Could you check a few things on this model? Use its own coordinates, in mm. Face numbers are marked on the shaded views. Give positions to 0.01 mm unless a question says otherwise; leave off trailing zeros. Write each loop counter-clockwise with the first axis right and the second up, starting at its lowest first coordinate (ties: lowest second). Pieces come first, ordered by that corner, then holes. Notation, with made-up numbers: (-37.5, 78.5) -> (-19.5, 78.5) arc R31 cw to (-19.5, 115.5) -> close; hole circle Ø11 at (-39, 36). An arc over 180 degrees is marked (long way). One line per question, with ' | ' between items.
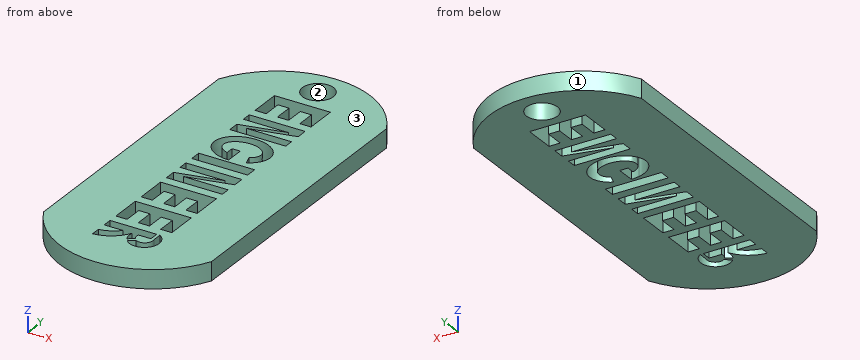
from build123d import *

# Parameters (mm, degrees)
F0_W     = 9
F0_H     = 1.8
F0_R     = 2.5
F0_W_2   = 0.5
F0_H_2   = 1.5
F1_DEPTH = 3


with BuildPart() as f1:
    # F0 (on Top) → F1 (new body)
    with BuildSketch(Plane.XY):
        with BuildLine():
            ThreePointArc((27, 0), (13.5, 8.4616515847), (0, 0))
            Line((0, 0), (0, -45))
            ThreePointArc((0, -45), (13.5, -53.4616515847), (27, -45))
            Line((27, -45), (27, 0))
        make_face()
        with BuildLine():
            Line((9, -43.8), (9, -42.3))
            Line((9, -42.3), (16.5, -42.3))
            Line((16.5, -42.3), (17, -42.3))
            ThreePointArc((17, -42.3), (17.66899179, -45.8750933579), (14.0327498007, -45.9562520189))
            ThreePointArc((14.0327498007, -45.9562520189), (13.8765268876, -45.76063274), (13.7416614246, -45.5497208918))
            ThreePointArc((13.7416614246, -45.5497208918), (13.452948616, -44.6980473592), (13.5, -43.8))
            ThreePointArc((13.5, -43.8), (11.6446119997, -45.8919179995), (9, -46.8))
            Line((9, -46.8), (9, -45.3))
            ThreePointArc((9, -45.3), (10.6342615319, -44.8185230639), (12, -43.8))
            Line((12, -43.8), (9, -43.8))
        make_face(mode=Mode.SUBTRACT)
        Polygon((9, -35.8), (18, -35.8), (18, -40.8), (16.2, -40.8), (16.2, -37.8), (14.4, -37.8), (14.4, -40.8), (12.6, -40.8), (12.6, -37.8), (10.8, -37.8), (10.8, -40.8), (9, -40.8), align=None, mode=Mode.SUBTRACT)
        Polygon((9, -34.3), (9, -29.3), (18, -29.3), (18, -34.3), (16.2, -34.3), (16.2, -31.3), (14.4, -31.3), (14.4, -34.3), (12.6, -34.3), (12.6, -31.3), (10.8, -31.3), (10.8, -34.3), align=None, mode=Mode.SUBTRACT)
        Polygon((9, -24.3), (9, -22.8), (18, -22.8), (18, -24.6), (10.779, -26.3), (18, -26.3), (18, -27.8), (9, -27.8), (9, -26), (16.2212999509, -24.3), align=None, mode=Mode.SUBTRACT)
        with Locations((13.5, -20.4)):
            Rectangle(F0_W, F0_H, mode=Mode.SUBTRACT)
        with BuildLine():
            add(Edge.make_bspline(
                [(18, -15.5), (18, -8.5693256297), (10.8288359741, -12.6833185304), (3.6576719482, -16.7973114311), (12.1711632237, -18.8439192062)],
                knots=[0, 0, 0, 2.2063112748, 2.2063112748, 4.4126225496, 4.4126225496, 4.4126225496], degree=2, weights=[1, 0.4507815404, 1, 0.4507815404, 1]))
            add(Edge.make_bspline(
                [(16, -18.4101779675), (18, -17.3708286934), (18, -15.5)],
                knots=[5.3014199506, 5.3014199506, 5.3014199506, 6.2831853072, 6.2831853072, 6.2831853072], degree=2, weights=[1, 0.8819171037, 1]))
            add(Edge.make_bspline(
                [(13.5, -19), (14.8650167038, -19), (16, -18.4101779675)],
                knots=[4.7123889804, 4.7123889804, 4.7123889804, 5.3014199506, 5.3014199506, 5.3014199506], degree=2, weights=[1, 0.9569428978, 1]))
            add(Edge.make_bspline(
                [(12.1711632237, -18.8439192062), (12.8204290441, -19), (13.5, -19)],
                knots=[4.4126225496, 4.4126225496, 4.4126225496, 4.7123889804, 4.7123889804, 4.7123889804], degree=2, weights=[1, 0.9887885233, 1]))
        make_face(mode=Mode.SUBTRACT)
        Polygon((9, -8), (9, -6.5), (18, -6.5), (18, -8.3), (10.779, -10), (18, -10), (18, -11.5), (9, -11.5), (9, -9.7), (16.2212999509, -8), align=None, mode=Mode.SUBTRACT)
        Polygon((9, -5), (9, 0), (18, 0), (18, -5), (16.2, -5), (16.2, -2), (14.4, -2), (14.4, -5), (12.6, -5), (12.6, -2), (10.8, -2), (10.8, -5), align=None, mode=Mode.SUBTRACT)
        with Locations((13.5, 3.9957081899)):
            Circle(F0_R, mode=Mode.SUBTRACT)
        with BuildLine():
            add(Edge.make_bspline(
                [(16.5, -15.5), (16.5, -11.9027200979), (11.9167297023, -13.8012089051), (7.3334594046, -15.6996977122), (12.1711632237, -17.2930969884)],
                knots=[0, 0, 0, 2.1267537417, 2.1267537417, 4.2535074833, 4.2535074833, 4.2535074833], degree=2, weights=[1, 0.4859234683, 1, 0.4859234683, 1]))
            Line((12.1711632237, -17.2930969884), (12.1711632237, -16))
            Line((12.1711632237, -16), (13.5, -16))
            Line((13.5, -16), (13.5, -17.5))
            add(Edge.make_bspline(
                [(13.5, -17.5), (14.6458980338, -17.5), (15.5, -16.990711985)],
                knots=[4.7123889804, 4.7123889804, 4.7123889804, 5.4421166366, 5.4421166366, 5.4421166366], degree=2, weights=[1, 0.934172359, 1]))
            add(Edge.make_bspline(
                [(15.5, -16.990711985), (16.5, -16.394427191), (16.5, -15.5)],
                knots=[5.4421166366, 5.4421166366, 5.4421166366, 6.2831853072, 6.2831853072, 6.2831853072], degree=2, weights=[1, 0.9128709292, 1]))
        make_face()
        with BuildLine():
            add(Edge.make_bspline(
                [(13.5, -19), (14.8650167038, -19), (16, -18.4101779675)],
                knots=[4.7123889804, 4.7123889804, 4.7123889804, 5.3014199506, 5.3014199506, 5.3014199506], degree=2, weights=[1, 0.9569428978, 1]))
            Line((16, -18.4101779675), (15.5, -16.990711985))
            add(Edge.make_bspline(
                [(13.5, -17.5), (14.6458980338, -17.5), (15.5, -16.990711985)],
                knots=[4.7123889804, 4.7123889804, 4.7123889804, 5.4421166366, 5.4421166366, 5.4421166366], degree=2, weights=[1, 0.934172359, 1]))
            Line((13.5, -17.5), (13.5, -19))
        make_face()
        with BuildLine():
            Line((17, -43.8), (16.5, -43.8))
            Line((16.5, -43.8), (14.5, -43.8))
            ThreePointArc((14.5, -43.8), (14.467921138, -44.3721848606), (14.6849938716, -44.9025658523))
            ThreePointArc((14.6849938716, -44.9025658523), (14.8482368669, -45.09345983), (15.0451432596, -45.2493978266))
            ThreePointArc((15.0451432596, -45.2493978266), (16.5242633972, -45.201349254), (17, -43.8))
        make_face()
        with Locations((16.75, -43.05)):
            Rectangle(F0_W_2, F0_H_2)
        with BuildLine():
            ThreePointArc((13.7416614246, -45.5497208918), (13.8765268876, -45.76063274), (14.0327498007, -45.9562520189))
            Line((14.0327498007, -45.9562520189), (15.0451432596, -45.2493978266))
            ThreePointArc((15.0451432596, -45.2493978266), (14.8482368669, -45.09345983), (14.6849938716, -44.9025658523))
            Line((14.6849938716, -44.9025658523), (13.7416614246, -45.5497208918))
        make_face()
    extrude(amount=F1_DEPTH)


solid = f1.part
Q1. Will these pins go through, and if not, where does the flat tip stop? pin 1 (1.4 mm diameter, centred on x = 11.5, z = 2, fed in from +Y); pin 2 (1.4 mm diameter, centred on x = 10, z = 2, fed in from +Y); pin 3 (0.9 mm diameter, centred on x = 9.5, z = 1, fed in from +Y).
Answer below:
pin 1: stops at y = 8.41 | pin 2: stops at y = 8.2 | pin 3: stops at y = 8.04
Q2. Imagine slicing it at A-A on y = -20.5. Please give me the cut outline in (x, z).
Answer below:
outline: (0, 0) -> (9, 0) -> (9, 3) -> (0, 3) -> close; (18, 0) -> (27, 0) -> (27, 3) -> (18, 3) -> close
Q3. Imagine slicing it at C-C on z = 1.75. Count the separate pieces of the cut face and the enclosed holes in it, and give its area (3 significant figures).
Answer below:
separate pieces: 1 | enclosed holes: 10 | area: 1,280 mm^2
Q4. Imagine slicing it at B-B on y = -43. Please give me the cut outline in (x, z).
Answer below:
outline: (0, 0) -> (9, 0) -> (9, 3) -> (0, 3) -> close; (16.5, 0) -> (17, 0) -> (17, 3) -> (16.5, 3) -> close; (17.77, 0) -> (27, 0) -> (27, 3) -> (17.77, 3) -> close
Q5. Imagine slicing it at D-D on y = 2.5. Please give me the cut outline in (x, z).
Answer below:
outline: (1.53, 0) -> (11.5, 0) -> (11.5, 3) -> (1.53, 3) -> close; (15.5, 0) -> (25.47, 0) -> (25.47, 3) -> (15.5, 3) -> close
Q6. If I drill on line 1 along X through (y, z) = (-39, 1.1); line 2 along X through (y, z) = (-20, 2.25); line 3 along X through (y, z) = (-17.5, 2.6), over which ranges is the centre line in solid material (lowest first)?
Answer below:
line 1: x = 0 to 9, 10.8 to 12.6, 14.4 to 16.2, 18 to 27 | line 2: x = 0 to 9, 18 to 27 | line 3: x = 0 to 9.81, 13.5 to 15.68, 17.19 to 27
Q7. If we mould it in two halves opening along X, with no side actions, what happens to the marked faces 1, 2 and 3? For each: +X half, -X half, draft (parallel to the pull), parting line (faces both ways), or undercut.
Answer below:
face 1: parting line | face 2: undercut | face 3: draft
